Could you check a few things on this model? Use its own coordinates, in mm. Coordinates: 2 decimals unless noted, no trailing zeros. Loops run counter-clockwise (first coordinate to the right, second up) from the corner with the lowest first, then second, coordinate; pieces in that order, holes last.
1) Imagine slicing it at A-A on x = -188.5. Please give me the cut outline in (y, z), plus the area to 3 significant figures.
2) Imagine slicing it at B-B on z = 95.5. Please give me the cut outline in (x, y).
3) Will these pins go through, and if not, where does the flat tip stop? P1, Ø2.5, axis at x = -109.5, y = -2.5, coming from the +Z side; P2, Ø1.5, axis at x = -47, y = -3, coming from the -Z side; P3, Ø1.5, axis at y = -3, z = -3, coming from the +X side.
4) Imagine slicing it at D-D on x = -50. Please give me the cut outline in (y, z), plus the area to 3 significant figures.
5) If I drill on line 1 along X through (y, z) = (-4.8, 135); line 2 along Z through (x, y) = (-78.5, -4.75); line 3 along Z through (x, y) = (-152, -3.1), over which ranges is the centre line in solid material (lowest first)?
6) Imagine slicing it at C-C on x = -131. Please give me the cut outline in (y, z), plus the area to 3 significant figures.
```python
from build123d import *

# Parameters (mm, degrees)
F0_W     = 15
F0_H     = 5.08
F1_DEPTH = 5.08
F2_DEPTH = 25
F4_DEPTH = 58
F5_W     = 15
F5_H     = 5.08
F6_DEPTH = 5.08


# Not quite as in the source:
# - a feature names something its author has since deleted; it is built from what else it names


with BuildPart() as f1:
    # F0 (on Front) → F1 (new body)
    with BuildSketch(Plane.XZ):
        Polygon((-87.5, 0), (-32.419, 0), (-32.419, 50), (-116.5, 50), (-144.9023774395, 50), (-196.5, 50), (-196.5, 101.5976225605), (-196.5, 130), (-246.5, 130), (-246.5, 0), (-231.5, 0), (-222.5, 0), (-207.5, 0), (-198.5, 0), (-183.5, 0), (-174.5, 0), (-159.5, 0), (-150.5, 0), (-135.5, 0), (-126.5, 0), (-111.5, 0), (-102.5, 0), align=None)
        with Locations((-95, -2.54)):
            Rectangle(F0_W, F0_H)
        Polygon((-144.9023774395, 50), (-116.5, 50), (-196.5, 130), (-196.5, 101.5976225605), align=None)
        with Locations((-119, -2.54)):
            Rectangle(F0_W, F0_H)
        with Locations((-143, -2.54)):
            Rectangle(F0_W, F0_H)
        with Locations((-239, -2.54)):
            Rectangle(F0_W, F0_H)
        with Locations((-167, -2.54)):
            Rectangle(F0_W, F0_H)
        with Locations((-215, -2.54)):
            Rectangle(F0_W, F0_H)
        with Locations((-191, -2.54)):
            Rectangle(F0_W, F0_H)
    extrude(amount=F1_DEPTH)

    # F2 (add): a face of the model
    f2_faces = [f1.faces().sort_by_distance(p)[0] for p in [
        (-221.5, -2.54, 130),
    ]]
    extrude(f2_faces, amount=F2_DEPTH)

    # F3 (on face) → F4 (cut)
    with BuildSketch(Plane(origin=(0, 0, 0), x_dir=(1, 0, 0), z_dir=(0, 0, -1))):
        Polygon((-32.419, 0), (-32.419, 5.08), (-35.3519393675, 0), align=None)
    extrude(amount=-F4_DEPTH, mode=Mode.SUBTRACT)

    # F5 (on face) → F6 (join)
    with BuildSketch(Plane.XY.offset(50)):
        with Locations((-94, -2.54)):
            Rectangle(F5_W, F5_H)
    extrude(amount=F6_DEPTH)


solid = f1.part
```
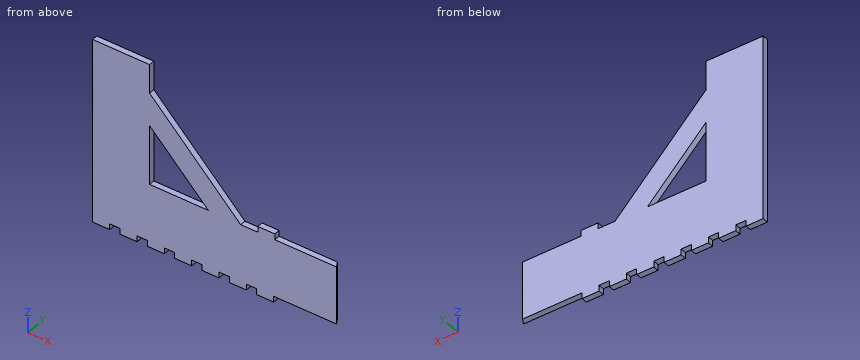
Filled in:
1. outline: (-5.08, -5.08) - (0, -5.08) - (0, 50) - (-5.08, 50) - close; (-5.08, 93.6) - (0, 93.6) - (0, 122) - (-5.08, 122) - close
1. area: 424 mm2
2. outline: (-246.5, -5.08) - (-196.5, -5.08) - (-196.5, 0) - (-246.5, 0) - close; (-190.4, -5.08) - (-162, -5.08) - (-162, 0) - (-190.4, 0) - close
3. P1: stops at z = 50
3. P2: stops at z = 0
3. P3: stops at x = -87.5
4. outline: (-5.08, 0) - (0, 0) - (0, 50) - (-5.08, 50) - close
4. area: 254 mm2
5. line 1: x = -246.5 to -196.5
5. line 2: z = 0 to 50
5. line 3: z = 0 to 50, 57.1 to 85.5
6. outline: (-5.08, 0) - (0, 0) - (0, 64.5) - (-5.08, 64.5) - close
6. area: 328 mm2
